The listing builds one solid part. Answer for the finished solid, in the listing's coordinates (mm). A direction names the side the tool comes from. Give positions to 0.01 mm unless a question says otherwise; leave off trailing zeros. Order: outer loops, then holes, each group sorted by start corner. A loop starts at its lowest first (then second) coordinate and runs counter-clockwise, first axis right, second up. Notation, with made-up numbers: (2, 39.5) - (27, 39.5) arc R23 cw to (27, 56.5) - close; hole circle Ø6 at (85.5, 7.5). An arc over 180 degrees is marked (long way). Answer in a Markdown table with one row per item.
from build123d import *

# Parameters (mm, degrees)
SKETCH017_W      = 20
SKETCH017_H      = 20
EXTRUDE016_DEPTH = 15
EXTRUDE017_DEPTH = 135


with BuildPart() as extrude016:
    # Sketch017 (on Face2 of Extrude017) → Extrude016 (new body, symmetric)
    with BuildSketch(Plane.XY.offset(81)):
        with Locations((0, 454.863156)):
            Rectangle(SKETCH017_W, SKETCH017_H)
    extrude(amount=EXTRUDE016_DEPTH, both=True)


with BuildPart() as u069:
    # Sketch019 (on Face6 of Extrude015) → Extrude017 (new body)
    with BuildSketch(Plane(origin=(0, 349.863156, 0), x_dir=(-1, 0, 0), z_dir=(0, 1, 0))):
        with BuildLine():
            Line((-32.5, 39), (-32.5, 81))
            Line((-32.5, 81), (32.5, 81))
            Line((32.5, 81), (32.5, 39))
            ThreePointArc((28.55865, 42.317536), (29.924137, 39.939783), (32.5, 39))
            Line((23.890032, 69.27962), (28.55865, 42.317536))
            ThreePointArc((23.890032, 69.27962), (21.329744, 73.737907), (16.5, 75.5))
            Line((-16.5, 75.5), (16.5, 75.5))
            ThreePointArc((-16.5, 75.5), (-21.329744, 73.737907), (-23.890032, 69.27962))
            Line((-23.890032, 69.27962), (-28.55865, 42.317536))
            ThreePointArc((-32.5, 39), (-29.924137, 39.939783), (-28.55865, 42.317536))
        make_face()
    extrude(amount=EXTRUDE017_DEPTH)

    # Cut006: cut Extrude016
    add(extrude016.part, mode=Mode.SUBTRACT)


solid = u069.part
Item 1: Determine the mould class of faces 4 (the face through (-29.89, 416.42, 39.97)), 5 (the face through (-3, 349.863, 76)), 6 (the face through (32.5, 416, 60)) for opening direction X: pulls with the +X half, pulls with the -X half, needs draft (parallel to the pull), parting line crosses it, or undercut.
Answer block:
| item | result |
|---|---|
| face 4 | undercut |
| face 5 | needs draft |
| face 6 | pulls with the +X half |
Item 2: Find section C-C on z = 47.5. Write down the section's boundary in (x, y).
Answer block:
| item | result |
|---|---|
| outline | (-32.5, 349.86) - (-27.66, 349.86) - (-27.66, 484.86) - (-32.5, 484.86) - close; (27.66, 349.86) - (32.5, 349.86) - (32.5, 484.86) - (27.66, 484.86) - close |
Item 3: Consider line 1 (X direction, y = 477, z = 49.5); line 2 (Z direction, x = 14.5, y = 458); line 3 (X direction, y = 461, z = 50). Determine where each line is inside the solid, lowest interval first.
Answer block:
| item | result |
|---|---|
| line 1 | -32.5 to -27.31, 27.31 to 32.5 |
| line 2 | 75.5 to 81 |
| line 3 | -32.5 to -27.23, 27.23 to 32.5 |
Item 4: Find section D-D on z = 78. Write down the section's boundary in (x, y), then the cut area to 4 significant figures.
Answer block:
| item | result |
|---|---|
| outline | (-32.5, 349.86) - (32.5, 349.86) - (32.5, 484.86) - (-32.5, 484.86) - close; hole (-10, 444.86) - (10, 444.86) - (10, 464.86) - (-10, 464.86) - close |
| area | 8,375 mm² |
Item 5: Which of the six approach directions +Z, -Z, +X, -X, +Y, -Y give full straight-line access (tool end or side, diameter ignored) to faces 1 (the face through (-3, 484.863, 76)), 2 (the face through (21, 416, 74)), 3 (the face through (0, 444.863, 78))?
Answer block:
| item | result |
|---|---|
| face 1 | +Z, -Z, +X, -X, +Y |
| face 2 | -Z, +Y, -Y |
| face 3 | +Z, -Z |
Item 6: Find section A-A on x = 8. Write down the section's boundary in (y, z).
Answer block:
| item | result |
|---|---|
| outline | (349.86, 75.5) - (444.86, 75.5) - (444.86, 81) - (349.86, 81) - close; (464.86, 75.5) - (484.86, 75.5) - (484.86, 81) - (464.86, 81) - close |
Item 7: This flat-tipped pin is pushed along its axis until it touches: P1, Ø4, axis at x = 3.5, y = 393, coming from the -Z side. Where does it stop, or does it pass through?
Answer block:
| item | result |
|---|---|
| P1 | z = 75.5 |
Item 8: Find section B-B on y = 432.5. Write down the section's boundary in (x, z), then the cut area to 3 significant figures.
Answer block:
| item | result |
|---|---|
| outline | (-32.5, 39) arc R4 ccw to (-28.56, 42.32) - (-23.89, 69.28) arc R7.5 cw to (-16.5, 75.5) - (16.5, 75.5) arc R7.5 cw to (23.89, 69.28) - (28.56, 42.32) arc R4 ccw to (32.5, 39) - (32.5, 81) - (-32.5, 81) - close |
| area | 845 mm² |
